Design review of the part built by this model. Coordinates are the model's own, in mm. A direction names the side the tool comes from. Round coordinates to 2 decimals unless told otherwise and drop trailing zeros. Order: outer loops, then holes, each group sorted by start corner. A loop starts at its lowest first (then second) coordinate and runs counter-clockwise, first axis right, second up. Notation, with made-up numbers: (-9, 20) - (33, 20) arc R30 ccw to (33, 45) - close; hole circle Ø3 at (-18, 35.5). An arc over 180 degrees is marked (long way). Write item = value, one per line.
from build123d import *

# Parameters (mm, degrees)
SKETCH1_R           = 30.48
SKETCH1_R_2         = 6.35
SKETCH1_R_3         = 2.54
BOSS_EXTRUDE1_DEPTH = 12.7
SKETCH2_OUTSIDE_W   = 80.934
SKETCH2_OUTSIDE_H   = 80.934
SKETCH2_OUTSIDE_R   = 17.3355
CUT_EXTRUDE1_DEPTH  = 20.828


with BuildPart() as part:
    # Sketch1 → Boss-Extrude1 (new body, symmetric)
    with BuildSketch(Plane(origin=(0, 0, 0), x_dir=(0, 0, -1), z_dir=(1, 0, 0))):
        Circle(SKETCH1_R)
        Circle(SKETCH1_R_2, mode=Mode.SUBTRACT)
        with Locations((0, 23.8125)):
            Circle(SKETCH1_R_3, mode=Mode.SUBTRACT)
        with Locations((20.622229928, 11.90625)):
            Circle(SKETCH1_R_3, mode=Mode.SUBTRACT)
        with Locations((20.622229928, -11.90625)):
            Circle(SKETCH1_R_3, mode=Mode.SUBTRACT)
        with Locations((0, -23.8125)):
            Circle(SKETCH1_R_3, mode=Mode.SUBTRACT)
        with Locations((-20.622229928, -11.90625)):
            Circle(SKETCH1_R_3, mode=Mode.SUBTRACT)
        with Locations((-20.622229928, 11.90625)):
            Circle(SKETCH1_R_3, mode=Mode.SUBTRACT)
    extrude(amount=BOSS_EXTRUDE1_DEPTH, both=True)

    # Sketch2 outside → Cut-Extrude1 (cut)
    with BuildSketch(Plane(origin=(12.7, 0, 0), x_dir=(0, 0, -1), z_dir=(1, 0, 0))):
        Rectangle(SKETCH2_OUTSIDE_W, SKETCH2_OUTSIDE_H)
        Circle(SKETCH2_OUTSIDE_R, mode=Mode.SUBTRACT)
    extrude(amount=-CUT_EXTRUDE1_DEPTH, mode=Mode.SUBTRACT)


solid = part.part
Item 1: Take a section at C-C, the plane x = -9.25. State the section outline as (y, z) points.
Data:
outline = circle Ø60.96 at (0, 0); hole circle Ø5.08 at (-23.81, 0); hole circle Ø5.08 at (-11.91, -20.62); hole circle Ø5.08 at (-11.91, 20.62); hole circle Ø12.7 at (0, 0); hole circle Ø5.08 at (11.91, -20.62); hole circle Ø5.08 at (11.91, 20.62); hole circle Ø5.08 at (23.81, 0)
Item 2: Take a section at A-A, the plane y = 0. State the section outline as (x, z) points.
Data:
outline = (-12.7, -30.48) - (-8.13, -30.48) - (-8.13, -17.34) - (12.7, -17.34) - (12.7, -6.35) - (-12.7, -6.35) - close; (-12.7, 6.35) - (12.7, 6.35) - (12.7, 17.34) - (-8.13, 17.34) - (-8.13, 30.48) - (-12.7, 30.48) - close
Item 3: For line 1 along Y through (x, z) = (-11.4, 0); line 2 along Y through (x, z) = (-8.5, 18.5); line 3 along Y through (x, z) = (-0.5, 0), list the stretches that pass through material, from the lowest coordinate up. Write a range as [from, to].
Data:
line_1 = [-30.48, -26.35], [-21.27, -6.35], [6.35, 21.27], [26.35, 30.48]
line_2 = [-24.22, -13.3], [-10.51, 10.51], [13.3, 24.22]
line_3 = [-17.34, -6.35], [6.35, 17.34]
Item 4: Take a section at B-B, the plane z = 0. State the section outline as (x, y) points.
Data:
outline = (-12.7, -30.48) - (-8.13, -30.48) - (-8.13, -26.35) - (-12.7, -26.35) - close; (-12.7, -21.27) - (-8.13, -21.27) - (-8.13, -17.34) - (12.7, -17.34) - (12.7, -6.35) - (-12.7, -6.35) - close; (-12.7, 6.35) - (12.7, 6.35) - (12.7, 17.34) - (-8.13, 17.34) - (-8.13, 21.27) - (-12.7, 21.27) - close; (-12.7, 26.35) - (-8.13, 26.35) - (-8.13, 30.48) - (-12.7, 30.48) - close
Item 5: Insertion check: P1, Ø8, axis at y = -23.81, z = 0, coming from the +X side; P2, Ø8, axis at x = 4.5, z = 9, coming from the +Y side; P3, Ø16.5, axis at y = 0, z = 0, coming from the -X side; P4, Ø4, axis at x = 2, y = -7, coming from the -Z side. Each pin has a flat end and moves straight along its axis. Give the tip position at first contact, or say it passes through.
Data:
P1 = -8.13
P2 = 16.6
P3 = -12.7
P4 = -16.6
Item 6: The part is to be moulded in two halves that separate along Z. For faces 1 (the face through (-10.446, -26.066, -1.172)), 2 (the face through (12.7, 0, -7)), 3 (the face through (-10.446, -12.879, 18.276)), 4 (the face through (2.43, 0.76, 17.32)), say which applies: +Z half, -Z half, draft (parallel to the pull), parting line (faces both ways), or undercut.
Data:
face_1 = undercut
face_2 = draft
face_3 = undercut
face_4 = parting line
Item 7: For faces 5 (the face through (-10.382, -29.755, 6.607)), 6 (the face through (-8.128, -13, -13)), list the 3-axis set-ups (+Z, -Z, +X, -X, +Y, -Y) from which the entire face can be reached by the end or side of a thin tool; tool diameter is ignored.
Data:
face_5 = +X, -X
face_6 = +X
Item 8: Take a section at D-D, the plane x = 6. State the section outline as (y, z) points.
Data:
outline = circle Ø34.67 at (0, 0); hole circle Ø12.7 at (0, 0)
